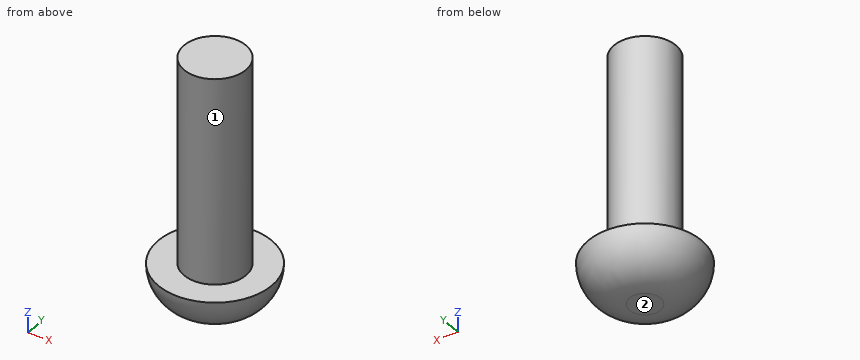
Autodesk Inventor part; units mm, degrees
ref_plane "YZ Plane" through (0, 0, 0) normal (1, 0, 0) x (0, 1, 0)
ref_plane "XZ Plane" through (0, 0, 0) normal (0, 1, 0) x (-1, 0, 0)
ref_plane "XY Plane" through (0, 0, 0) normal (0, 0, 1) x (1, 0, 0)
sketch "スケッチ1" plane through (0, 0, 0) normal (0, 0, 1) x (1, 0, 0)
  circle A0 centre (0, 0) radius 1.5
  dimension "d0" = 3
extrude "押し出し1" add sketch "スケッチ1" along normal blind 10
sketch "スケッチ2" plane through (0, 0, 0) normal (0, 0, -1) x (-1, 0, 0)
  circle A0 centre (0, 0) radius 2.75
  dimension "d3" = 5.5
extrude "押し出し2" add sketch "スケッチ2" along normal blind 2
fillet "フィレット1" radius 2 1 edges at (2.75, 0, -2)
thread "ねじ1"
properties part number "ネジm3,10" material "鋼、高強度、低合金"
The listing builds one solid part. Answer for the finished solid, in the listing's coordinates (mm). Face numbers are marked on the shaded views. A direction names the side the tool comes from. Give positions to 0.01 mm unless a question says otherwise; leave off trailing zeros. Order: outer loops, then holes, each group sorted by start corner. A loop starts at its lowest first (then second) coordinate and runs counter-clockwise, first axis right, second up. Notation, with made-up numbers: (39.25, -15) -> (97.25, -15) arc R28 cw to (97.25, 6) -> close; hole circle Ø8 at (19, 36). An arc over 180 degrees is marked (long way). Answer as a JSON object with one key per item and string values. Group by question number.
Item 1: Flat-ended cylindrical pins translate along their axes: pin 1 (1.5 mm diameter, centred on x = 1, z = -1, fed in from -Y); pin 2 (1.5 mm diameter, centred on x = 0, y = -2, fed in from +Z); pin 3 (1 mm diameter, centred on x = 1, z = 2.5, fed in from +Y). Find the tip coordinate at first contact, or state that the pin passes through.
Item 2: The part is cut by section A-A on z = 6. Write down the section's boundary in (x, y), and give its area (3 significant figures).
Item 3: Consider L1, parallel to Y at x = 0.1, z = 7.75; L2, parallel to X at y = 0.55, z = 1.75; L3, parallel to Y at x = 1, z = 2. Determine where each line is inside the solid, lowest interval first. Write a range as from..to.
Item 4: A tool of negligible diameter and unlimited length cuts with its end or side. For the marked faces 1 and 2, from which of +Z, -Z, +X, -X, +Y, -Y can it reach the whole face along a straight path? Write none if from no direction.
Result set:
{
 "1": {"pin 1": "y = -2.65", "pin 2": "z = 10", "pin 3": "y = 1.41"},
 "2": {"outline": "circle Ø3 at (0, 0)", "area": "7.07 mm²"},
 "3": {"L1": "-1.5..1.5", "L2": "-1.4..1.4", "L3": "-1.12..1.12"},
 "4": {"face 1": "+Z", "face 2": "-Z, +X, -X, +Y, -Y"}
}
